Geometry: final body of the model. Coordinates: model frame, mm. Coordinates: 2 decimals unless noted, no trailing zeros. Write each loop counter-clockwise with the first axis right and the second up, starting at its lowest first coordinate (ties: lowest second). Pieces come first, ordered by that corner, then holes.
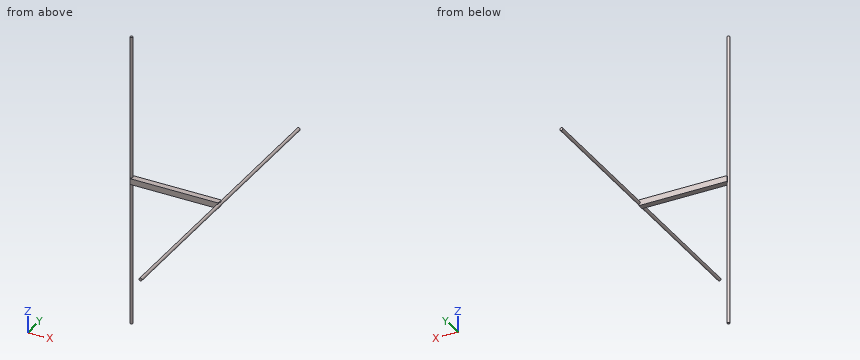
from build123d import *

# Parameters (mm, degrees)
F3_R     = 0.5
F4_DEPTH = 50
F5_R     = 0.5
F6_DEPTH = 50
F7_W     = 2
F7_H     = 2
F8_DEPTH = 30


with BuildPart() as f4:
    # F3 (on Front) → F4 (new body, symmetric)
    with BuildSketch(Plane.XZ):
        Circle(F3_R)
    extrude(amount=F4_DEPTH, both=True)



with BuildPart() as f6:
    # F5 (on Top) → F6 (new body, symmetric)
    with BuildSketch(Plane.XY):
        with Locations((-30, 0)):
            Circle(F5_R)
    extrude(amount=F6_DEPTH, both=True)


with BuildPart() as f4_1:
    add(f4.part)

    add(f6.part)  # F8 merges F6
    # F7 (on Right) → F8 (join)
    with BuildSketch(Plane.YZ):
        Rectangle(F7_W, F7_H)
    extrude(amount=-F8_DEPTH)


solid = f4_1.part
Item 1: Section A-A, the plane y = 16. Output: boundary loops of the cut face in (x, z), plus the area to 3 significant figures.
Derived:
outline: circle Ø1 at (0, 0)
area: 0.785 mm2
Item 2: Section B-B, the plane z = -16. Output: boundary loops of the cut face in (x, y).
Derived:
outline: circle Ø1 at (-30, 0)
Item 3: Pin query (flat end, axial travel): pin 1 (1.6 mm diameter, centred on x = -11, y = 0, fed in from -Z); pin 2 (1.6 mm diameter, centred on x = -13, z = 0, fed in from -Y); pin 3 (1 mm diameter, centred on x = -15, z = 0, fed in from +Y); pin 4 (6 mm diameter, centred on x = -26, z = 37.5, fed in from -Y). Return the tip coordinate at first contact, or that it passes through.
Derived:
pin 1: stops at z = -1
pin 2: stops at y = -1
pin 3: stops at y = 1
pin 4: passes through
Item 4: Section C-C, the plane x = -12.5. Output: boundary loops of the cut face in (y, z), plus the area to 3 significant figures.
Derived:
outline: (-1, -1) - (1, -1) - (1, 1) - (-1, 1) - close
area: 4.00 mm2
